Part model, mm, in its own coordinate system. Give positions to 0.01 mm unless a question says otherwise; leave off trailing zeros. Write each loop counter-clockwise with the first axis right and the second up, starting at its lowest first coordinate (ties: lowest second). Pieces come first, ordered by that corner, then holes. Notation, with made-up numbers: M -38.5,88.5 L -33.5,88.5 A6 ccw -33.5,98.5 Z; hole C 8,15 d10. An arc over 180 degrees is marked long. Use a Markdown table: item, result. Add a question column.
from build123d import *

# Parameters (mm, degrees)
F0_R            = 9
F0_R_2          = 6
F1_DEPTH        = 240
F3_W            = 18
F3_H            = 240
F4_DEPTH        = 1.5
F4_COPIES_COUNT = 3


# Not quite as in the source:
# - a pattern or mirror of a feature is missing from the dataset's text; its kind, count and spacing are read off the source's solid


with BuildPart() as f1:
    # F0 (on Top) → F1 (new body)
    with BuildSketch(Plane.XY):
        Circle(F0_R)
        Circle(F0_R_2, mode=Mode.SUBTRACT)
    extrude(amount=F1_DEPTH)

    # F3 (on offset) → F4 (cut)
    with BuildSketch(Plane.XZ.offset(9)):
        with Locations((0, 120)):
            Rectangle(F3_W, F3_H)
    f4 = extrude(amount=-F4_DEPTH, mode=Mode.SUBTRACT)

    # F4_copies: F4 ×3 about axis
    f4_copies_axis = Axis((0, 0, 0), (0, 0, 1))
    for i in range(1, F4_COPIES_COUNT):
        add(f4.rotate(f4_copies_axis, i * 360 / F4_COPIES_COUNT), mode=Mode.SUBTRACT)


solid = f1.part
1. Drill centre lines: probe 1 along Y at (x, z) = (0.75, 121); probe 2 along Y at (x, z) = (3.25, 101.5); probe 3 along X at (y, z) = (4.75, 133). Where is each one in solid material? Low to high. Write a range as [from, to].
2. Cut at A-A (x = 0). Write the cut outline in (y, z), then the cut area to 3 significant figures.
3. Flat gauge pins, fed straight in: pin 1 (8 mm diameter, centred on y = 4, z = 170, fed in from +X); pin 2 (4 mm diameter, centred on x = -3.5, z = 25.5, fed in from +Y); pin 3 (2 mm diameter, centred on y = 1.5, z = 183, fed in from +X). Where does each tip first touch, or does it go through?
4. Mould opens along Y. For faces 1 (the flat face through (-6.1, -1, 0)), 2 (the flat face through (-6.46, 3.81, 121.68)), 3 (the cylindrical face through (-6, 0, 118)) say: released by +Y, released by -Y, zero draft, split by the parting line, or undercut.
5. Cut at B-B (z = 157). Write the cut outline in (x, y).
A:
| question | item | result |
|---|---|---|
| 1 | probe 1 | y = [-7.5, -5.95], [5.95, 8.97] |
| 1 | probe 2 | y = [-7.5, -5.04], [5.04, 8.39] |
| 1 | probe 3 | x = [-5.92, -3.67], [3.67, 5.92] |
| 2 | outline | M -7.5,0 L -6,0 L -6,240 L -7.5,240 Z; M 6,0 L 9,0 L 9,240 L 6,240 Z |
| 2 | area | 1,080 mm² |
| 3 | pin 1 | stops at x = 8.66 |
| 3 | pin 2 | stops at y = 8.87 |
| 3 | pin 3 | stops at x = 8.37 |
| 4 | face 1 | zero draft |
| 4 | face 2 | released by +Y |
| 4 | face 3 | undercut |
| 5 | outline | M -8.98,-0.56 A9 ccw -4.97,-7.5 L 4.97,-7.5 A9 ccw 8.98,-0.56 L 4.01,8.06 A9 ccw -4.01,8.06 Z; hole C 0,0 d12 |
